Autodesk Inventor part; units mm, degrees
ref_plane "YZ Plane" through (0, 0, 0) normal (1, 0, 0) x (0, 1, 0)
ref_plane "XZ Plane" through (0, 0, 0) normal (0, 1, 0) x (-1, 0, 0)
ref_plane "XY Plane" through (0, 0, 0) normal (0, 0, 1) x (1, 0, 0)
sketch "草图1" plane through (0, 0, 0) normal (0, 1, 0) x (-1, 0, 0)
  line L0 (0, 65) -> (-12, 65)
  line L1 (-12, 65) -> (-12, 38)
  line L2 (-12, 38) -> (-14.5, 38)
  line L3 (-14.5, 38) -> (-14.5, 40)
  line L4 (-14.5, 40) -> (-24, 40)
  line L5 (-24, 40) -> (-24, 38)
  line L6 (-24, 38) -> (-38, 38)
  line L7 (-38, 38) -> (-38, 0)
  line L8 (-38, 0) -> (0, 0)
  line L9 (0, 0) -> (0, 65)
  line L10 (0, 38) -> (-1, 37)
  line L11 (-1, 37) -> (-1, 0)
  line L12 (-38, 34) -> (-15, 31.6998)
  line L13 (-15, 31.6998) -> (-15, 0)
  line L14 (7.6, 0) -> (-45.6, 0)
  dimension "d2" = 65
  dimension "d4" = 26
  dimension "d5" = 12
  dimension "d6" = 40
  dimension "d7" = 38
  dimension "d8" = 12
  dimension "d9" = 2.5
  dimension "d10" = 38
  dimension "d11" = 45
  dimension "d12" = 1
  dimension "d13" = 15
  dimension "d14" = 34
  dimension "d15" = 84.289
revolve "旋转1" add sketch "草图1" angle 360 about axis through (-10, 0, 0) along (1, 0, 0) contours L9 L10 L11 L8 L13 L12 L7 L6 L5 L4 L3 L2 L1 L0
sketch "草图2" plane through (0, 0, 0) normal (0, 1, 0) x (-1, 0, 0)
  line L0 (-24, 38) -> (-38, 38)
  line L1 (-39, 38) -> (-32, 38)
  line L2 (-32, 38) -> (-32, -20)
  line L3 (-32, -20) -> (-39, -20)
  line L4 (-39, -20) -> (-39, 38)
  point P0 (0, 0)
  dimension "d17" = 7
extrude "拉伸1" cut sketch "草图2" along normal mid plane 8
sketch "草图3" plane through (0, 0, 0) normal (0, 0, 1) x (1, 0, 0)
  line L0 (38, 4) -> (38, 38)
  line L1 (24, -38) -> (38, -38)
  line L2 (38, 38) -> (31, 38)
  line L3 (31, 38) -> (31, -38)
  line L4 (31, -38) -> (38, -38)
  line L5 (38, -38) -> (38, 38)
  point P0 (0, 0)
  point P1 (38, -4)
  dimension "d20" = 7
extrude "拉伸2" cut sketch "草图3" along normal mid plane 8
sketch "草图4" plane through (0, 0, 0) normal (-1, 0, 0) x (0, 0, 1)
  circle A0 centre (37.1231, 37.1231) radius 5.5
  circle A1 centre (-37.1231, 37.1231) radius 5.5
  circle A2 centre (-37.1231, -37.1231) radius 5.5
  circle A3 centre (37.1231, -37.1231) radius 5.5
  line L0 (37.1231, 37.1231) -> (0, 0)
  line L1 (0, -91) -> (0, 91)
  dimension "d23" = 11
  dimension "d24" = 52.5
  dimension "d27" = 360
  dimension "d42" = 45
extrude "拉伸3" cut sketch "草图4" against normal up to surface (12 mm away)
chamfer "倒角1" distance 1 angle 45 1 edges at (0, 0, -65)
fillet "圆角1" radius 5 1 edges at (15, 0, -31.6998)
sketch "草图5" plane through (0, 0, 0) normal (0, 0, 1) x (1, 0, 0)
  line L0 (0, -38) -> (0, 38)
  line L1 (0, 23) -> (3.1405, 23)
  line L2 (3.1405, 23) -> (4, 30)
  line L3 (4, 30) -> (11, 30)
  line L4 (11, 30) -> (11.8595, 23)
  line L5 (11.8595, 23) -> (15, 23)
  line L6 (15, 27.1749) -> (15, -27.1749)
  line L7 (0, 23) -> (0, 0)
  line L8 (0, 0) -> (15, 0)
  line L9 (15, 23) -> (15, 0)
  line L10 (-3, 0) -> (18, 0)
  point P0 (7.5, 30)
  dimension "d35" = 23
  dimension "d36" = 30
  dimension "d37" = 7
  dimension "d38" = 7
  dimension "d39" = 7
  dimension "d40" = 7.5
revolve "旋转2" cut sketch "草图5" angle 360 about axis through (-10, 0, 0) along (1, 0, 0)
equation "\"d2\" = 0.5 * D2"
equation "\"d4\" = M"
equation "\"d5\" = e"
equation "\"d6\" = 0.5 * D"
equation "\"d7\" = 0.5 * D_d"
equation "\"d8\" = e1"
equation "\"d10\" = 0.5 * D_d"
equation "\"d13\" = b1"
equation "\"d14\" = 0.5 * D4"
equation "\"d17\" = h_b"
equation "\"d18\" = b"
equation "\"d20\" = h_b"
equation "\"d21\" = b"
equation "\"d23\" = d0"
equation "\"d24\" = 0.5 * D0"
equation "\"d29\" = b"
equation "\"d35\" = 0.5 * d1"
equation "\"d36\" = 0.5 * d1_D0"
equation "\"d37\" = d1_b"
equation "\"d0\" = 11"
equation "\"D0\" = 105"
equation "\"D4\" = 68"
equation "\"D_d\" = 76"
equation "\"e\" = 12"
equation "\"e1\" = 12"
equation "\"b\" = 8"
equation "\"h_b\" = 7"
equation "\"M\" = 26"
equation "\"b1\" = 15"
equation "\"d1\" = 46"
equation "\"d1_b\" = 7"
properties part number "低速轴承透盖" material "灰口铁"
Could you check a few things on this model? Use its own coordinates, in mm. A direction names the side the tool comes from. Round coordinates to 2 decimals unless told otherwise and drop trailing zeros. Order: outer loops, then holes, each group sorted by start corner. A loop starts at its lowest first (then second) coordinate and runs counter-clockwise, first axis right, second up. Notation, with made-up numbers: M -7.5,67 L 7.5,67 A22 cw 7.5,80 Z; hole C 0.25,48.5 d1. An arc over 180 degrees is marked long. One line per question, with ' | ' between items. Start each with the question number.
(1) Thinking about a two-plate mould opening in Z: for faces 5 (the face through (38, -26, 25)), 6 (the face through (31.098, 33.713, 17.535)), 7 (the face through (5.9, -32.5, 40.1)), which applies, +Z half, -Z half, draft (parallel to the pull), parting line (faces both ways), or undercut?
(2) Please list where these lines run through material, in increasing order: line 1 along Z through (x, y) = (2.6, 0); line 2 along Y through (x, z) = (11.5, 42); line 3 along X through (y, z) = (11.5, -20).
(3) Suppose I cut it at B-B on x = 17. List the corners of the cut face in (y, z) for me, then the cut area to 3 significant figures.
(4) Suppose I cut it at C-C on x = 28.5. List the corners of the cut face in (y, z) for me, then the cut area to 3 significant figures.
(5) For faces 1 (the face through (24, 14.6, 35.4)), 2 (the face through (5.92, -31.67, -37.84)), 3 (the face through (34, 35, -4)), 4 (the face through (11.806, -5.081, 22.881)), which set-ups out of +Z, -Z, +X, -X, +Y, -Y let a thin tool reach every point of the face, with its end or its side?
(6) For P1, Ø1.5, axis at x = 13, y = -1.5, coming from the -Z side; P2, Ø4, axis at y = 2.5, z = -25, coming from the +X side; P3, Ø10, axis at y = 37.12, z = -37.12, coming from the -X side; P4, Ø1.5, axis at y = -34.5, z = -1, coming from the +X side, each with a flat end and sliding along its axis, tell me the tip position at first contact or that it passes through.
(7) Suppose I cut it at A-A on x = 9. List the corners of the cut face in (y, z) for me.
Geometry results:
1) face 5: draft | face 6: parting line | face 7: undercut
2) line 1: -65 to -23, 23 to 65 | line 2: -49.61 to -39.67, -34.58 to 34.58, 39.67 to 49.61 | line 3: 1 to 3.15, 11.85 to 15
3) outline: C 0,0 d80; hole C 0,0 d62.35 | area: 1,970 mm²
4) outline: C 0,0 d76; hole C 0,0 d66.1 | area: 1,100 mm²
5) face 1: +X | face 2: +X, -X | face 3: +X, +Y, -Y | face 4: none
6) P1: z = -37.99 | P2: x = 15 | P3: through | P4: x = 31
7) outline: C 0,0 d130; hole C -37.12,-37.12 d11; hole C -37.12,37.12 d11; hole C 0,0 d60; hole C 37.12,-37.12 d11; hole C 37.12,37.12 d11
